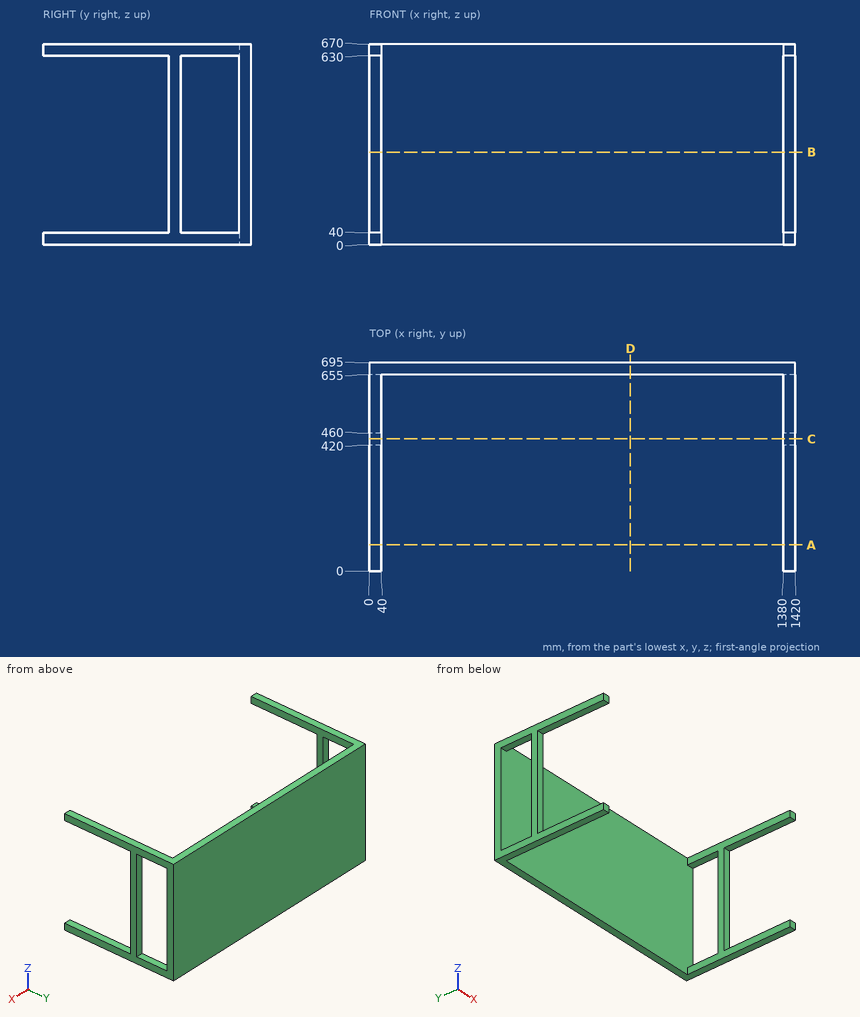
Study the drawing (mm; zero at the part's minimum x, y, z) and answer. Round coordinates to 2 decimals unless told otherwise and drop trailing zeros. Loops run counter-clockwise (first coordinate to the right, second up) from the corner with the lowest first, then second, coordinate; pieces in that order, holes last. Notation, with made-up numbers: (73.25, -1) -> (102.25, -1) arc R32 cw to (102.25, 31) -> close; hole circle Ø3 at (48, 20). An arc over 180 degrees is marked (long way). Use one line per item in the form item = value.
1. The part is cut by section C-C on y = 441. Determine the outline of the cut face in (x, z).
Answer key:
outline = (0, 0) -> (40, 0) -> (40, 670) -> (0, 670) -> close; (1380, 0) -> (1420, 0) -> (1420, 670) -> (1380, 670) -> close
2. The part is cut by section B-B on z = 309. Determine the outline of the cut face in (x, y).
Answer key:
outline = (0, 420) -> (40, 420) -> (40, 460) -> (0, 460) -> close; (0, 655) -> (1420, 655) -> (1420, 695) -> (0, 695) -> close; (1380, 420) -> (1420, 420) -> (1420, 460) -> (1380, 460) -> close
3. Find the intervals of material crossed by probe 1 along X at (y, z) = (449, 313); probe 2 along Y at (x, z) = (727.5, 625.5), in increasing order. Write a range as [from, to].
Answer key:
probe_1 = [0, 40], [1380, 1420]
probe_2 = [655, 695]
4. The part is cut by section D-D on x = 871. Determine the outline of the cut face in (y, z), and give its area (3 significant figures).
Answer key:
outline = (655, 0) -> (695, 0) -> (695, 670) -> (655, 670) -> close
area = 26,800 mm²
5. The part is cut by section A-A on y = 88. Determine the outline of the cut face in (x, z).
Answer key:
outline = (0, 0) -> (40, 0) -> (40, 40) -> (0, 40) -> close; (0, 630) -> (40, 630) -> (40, 670) -> (0, 670) -> close; (1380, 0) -> (1420, 0) -> (1420, 40) -> (1380, 40) -> close; (1380, 630) -> (1420, 630) -> (1420, 670) -> (1380, 670) -> close
6. Flat-ended cylindrical pins translate along their axes: pin 1 Ø20 at (x, z) = (1399.5, 305.5) entering from -Y; pin 2 Ø5 at (x, z) = (901, 127.5) entering from -Y. Find the tip coordinate at first contact, or state that the pin passes through.
Answer key:
pin_1 = 420
pin_2 = 655
